```python
from build123d import *

# Parameters (mm, degrees)
ESQUISSE2_W             = 187.693077266
ESQUISSE2_H             = 255.801785532
BOSS_EXTRU_1_DEPTH      = 10
ESQUISSE1_R             = 8.980927744
ENL_V_MAT_EXTRU_1_DEPTH = 1


with BuildPart() as part:
    # Esquisse2 → Boss.-Extru.1 (new body)
    with BuildSketch(Plane.XY):
        Rectangle(ESQUISSE2_W, ESQUISSE2_H)
    extrude(amount=-BOSS_EXTRU_1_DEPTH)

    # Esquisse1 → Enlèv. mat.-Extru.1 (cut)
    with BuildSketch(Plane.XY):
        with Locations((-14.068497164, 57.651010039)):
            Circle(ESQUISSE1_R)
        with BuildLine():
            Line((-18.438094574, -67.249269982), (0.561905426, -58.249269982))
            add(Edge.make_bspline(
                [(0.561905426, -58.249269982), (0.895238759, -55.249269982), (2.440765615, -52.136953462), (1.561905426, -49.249269982), (-0.003041236, -44.107302379), (-3.771427907, -39.915936649), (-6.438094574, -35.249269982)],
                knots=[0, 0, 0, 0, 1, 1, 1, 2, 2, 2, 2], degree=3))
            add(Edge.make_bspline(
                [(-6.438094574, -35.249269982), (-4.438094574, -32.582603316), (-3.287386291, -28.979197096), (-0.438094574, -27.249269982), (6.334594522, -23.137280174), (14.228572093, -21.249269982), (21.561905426, -18.249269982)],
                knots=[0, 0, 0, 0, 1, 1, 1, 2, 2, 2, 2], degree=3))
            Line((21.561905426, -18.249269982), (54.561905426, -18.249269982))
            Line((54.561905426, -18.249269982), (63.561905426, -24.249269982))
            Line((63.561905426, -24.249269982), (62.561905426, -33.249269982))
            add(Edge.make_bspline(
                [(62.561905426, -33.249269982), (54.348122416, -32.222547106), (39.619427755, -26.495850742), (33.561905426, -29.249269982), (26.906606899, -32.274405676), (20.228572093, -35.249269982), (13.561905426, -38.249269982)],
                knots=[0, 0, 0, 0, 1, 1, 1, 2, 2, 2, 2], degree=3))
            Line((13.561905426, -38.249269982), (14.561905426, -54.249269982))
            Line((14.561905426, -54.249269982), (38.561905426, -54.249269982))
            Line((38.561905426, -54.249269982), (39.561905426, -59.249269982))
            Line((39.561905426, -59.249269982), (15.561905426, -68.249269982))
            Line((15.561905426, -68.249269982), (13.561905426, -102.249269982))
            Line((13.561905426, -102.249269982), (5.561905426, -109.249269982))
            Line((5.561905426, -109.249269982), (1.561905426, -105.249269982))
            Line((1.561905426, -105.249269982), (7.561905426, -69.249269982))
            Line((7.561905426, -69.249269982), (-24.438094574, -87.249269982))
            Line((-24.438094574, -87.249269982), (-34.438094574, -75.249269982))
            Line((-34.438094574, -75.249269982), (-31.438094574, -30.249269982))
            add(Edge.make_bspline(
                [(-31.438094574, -30.249269982), (-37.438094574, -29.249269982), (-43.966600051, -29.906853036), (-49.438094574, -27.249269982), (-56.041298676, -24.041999418), (-60.771427907, -17.915936649), (-66.438094574, -13.249269982)],
                knots=[0, 0, 0, 0, 1, 1, 1, 2, 2, 2, 2], degree=3))
            add(Edge.make_bspline(
                [(-66.438094574, -13.249269982), (-66.104761241, -6.582603316), (-67.548913267, 0.418273938), (-65.438094574, 6.750730018), (-64.019958082, 11.005139495), (-59.438094574, 13.417396684), (-56.438094574, 16.750730018)],
                knots=[0, 0, 0, 0, 1, 1, 1, 2, 2, 2, 2], degree=3))
            Line((-56.438094574, 16.750730018), (-54.438094574, -9.249269982))
            Line((-54.438094574, -9.249269982), (-34.438094574, -20.249269982))
            add(Edge.make_bspline(
                [(-34.438094574, -20.249269982), (-33.104761241, -19.582603316), (-31.15649663, -19.555455539), (-30.438094574, -18.249269982), (-27.335628903, -12.608423308), (-25.771427907, -6.249269982), (-23.438094574, -0.249269982)],
                knots=[0, 0, 0, 0, 1, 1, 1, 2, 2, 2, 2], degree=3))
            Line((-23.438094574, -0.249269982), (-17.438094574, 0.750730018))
            Line((-17.438094574, 0.750730018), (-8.438094574, -13.249269982))
            add(Edge.make_bspline(
                [(-8.438094574, -13.249269982), (-4.438094574, -6.915936649), (1.193127025, -1.355605184), (3.561905426, 5.750730018), (8.39884273, 20.261541929), (-2.572357609, 24.518259979), (-11.438094574, 32.750730018)],
                knots=[0, 0, 0, 0, 1, 1, 1, 2, 2, 2, 2], degree=3))
            Line((-11.438094574, 32.750730018), (-30.438094574, 28.750730018))
            add(Edge.make_bspline(
                [(-30.438094574, 28.750730018), (-29.771427907, 31.417396684), (-30.565499704, 35.010125821), (-28.438094574, 36.750730018), (-22.669357465, 41.470605834), (-15.104761241, 43.417396684), (-8.438094574, 46.750730018), (-6.438094574, 47.750730018), (-4.667576181, 49.579231433), (-2.438094574, 49.750730018), (-0.018539167, 49.936849664), (2.228572093, 48.417396684), (4.561905426, 47.750730018)],
                knots=[0, 0, 0, 0, 1, 1, 1, 2, 2, 2, 3, 3, 3, 4, 4, 4, 4], degree=3))
            add(Edge.make_bspline(
                [(4.561905426, 47.750730018), (3.561905426, 44.084063351), (0.640128228, 40.437838809), (1.561905426, 36.750730018), (3.156422174, 30.372663025), (9.533684179, 26.004412197), (11.561905426, 19.750730018), (13.628861322, 13.377616005), (13.257677863, 6.443736403), (13.561905426, -0.249269982), (13.595750298, -0.99385717), (13.061974693, -1.696561846), (12.561905426, -2.249269982), (6.708744727, -8.71855286), (0.838084785, -15.189510601), (-5.438094574, -21.249269982), (-8.846299856, -24.539950945), (-14.599652494, -25.882970043), (-16.438094574, -30.249269982), (-25.647412644, -52.121400398), (-23.800738795, -52.948885392), (-18.438094574, -67.249269982)],
                knots=[0, 0, 0, 0, 1, 1, 1, 2, 2, 2, 3, 3, 3, 4, 4, 4, 5, 5, 5, 6, 6, 6, 7, 7, 7, 7], degree=3))
        make_face()
    extrude(amount=-ENL_V_MAT_EXTRU_1_DEPTH, mode=Mode.SUBTRACT)


solid = part.part
```
The model under review builds one solid part; all positions refer to its coordinate system, in mm. A direction names the side the tool comes from. Round coordinates to 2 decimals unless told otherwise and drop trailing zeros.
(1) Wall thickness on L1, parallel to Z at x = 32, y = -20.5; L2, parallel to X at y = 26.5, z = -0.75: over which ranges is each line inside the solid? List them lowest first.
(2) Mouldability with a two-part tool opening along X and no side actions: class faces 3 (the flat face through (93.847, -2, -5)), 4 (the flat face through (-44.58, -14.67, -0.49)), 5 (the flat face through (-93.847, -2, -5)), 6 (the flat face through (-1, 2, -10)) as +X half, -X half, draft (parallel to the pull), parting line (faces both ways), or undercut.
(3) Machinability: for faces 1 (the cylindrical face through (-5.502, 60.349, -0.493)), 2 (the flat face through (-1, 127.901, -5)), which of the approach directions +Z, -Z, +X, -X, +Y, -Y give a long, thin tool a straight path to every point of the face, cutting with its end or side? Answer none if there is none.
Findings below:
1. L1: z = -10 to -1
1. L2: x = -93.85 to -3.94, 7.7 to 93.85
2. face 3: +X half
2. face 4: undercut
2. face 5: -X half
2. face 6: draft
3. face 1: +Z
3. face 2: +Z, -Z, +X, -X, +Y
